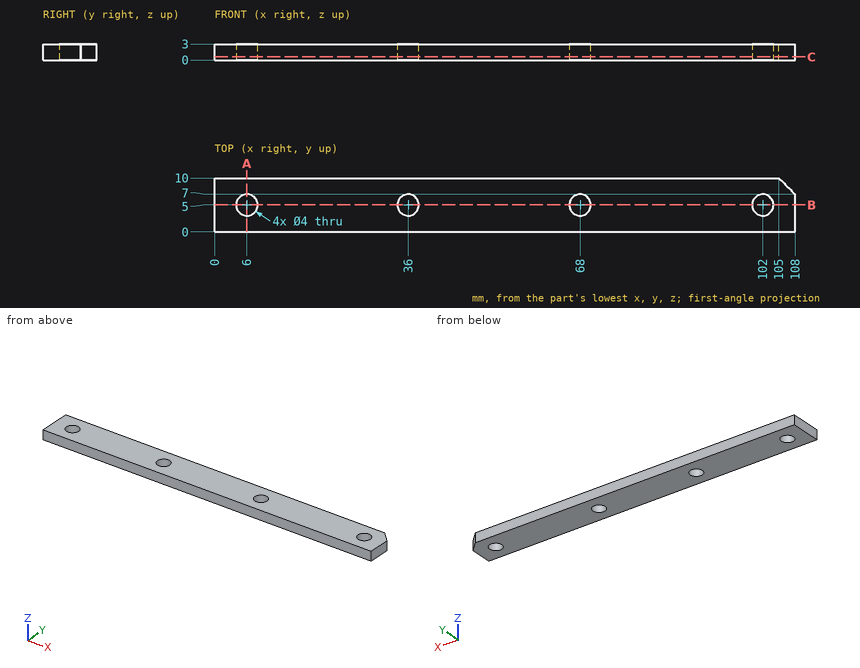
Job drawing, mm, ordinate dimensions from the low corner. One solid piece. Coordinates: 2 decimals unless noted, no trailing zeros. Order: outer loops, then holes, each group sorted by start corner. A loop starts at its lowest first (then second) coordinate and runs counter-clockwise, first axis right, second up. Notation, with made-up numbers: (10.25, 24) -> (17.25, 24) arc R30 cw to (17.25, 63) -> close; hole circle Ø11 at (-24.5, 56.5). An arc over 180 degrees is marked (long way). Put each result on its own line as item: value. Start each with the question number.
(1) Pin check, flat tip, straight feed: pin 1 Ø2.5 at (x, y) = (36, 5) entering from +Z. Stop position of the tip, or through.
(2) Band-saw the part on A-A (x = 6). Give the cut face in (y, z).
(3) Band-saw the part on C-C (z = 0.6). Give the cut face in (x, y), then the cut area to 3 significant figures.
(4) Band-saw the part on B-B (y = 5). Give the cut face in (x, z).
(5) Probe line 1 along X through (y, z) = (5.25, 2.55); line 2 along Y through (x, z) = (6, 2); line 3 along X through (y, z) = (6.5, 2.05). List the from-to ranges inside material, lowest first. Write a range as [from, to].
Determined:
1. pin 1: passes through
2. outline: (0, 0) -> (3, 0) -> (3, 3) -> (0, 3) -> close; (7, 0) -> (10, 0) -> (10, 3) -> (7, 3) -> close
3. outline: (0, 0) -> (108, 0) -> (108, 7) -> (105, 10) -> (0, 10) -> close; hole circle Ø4 at (6, 5); hole circle Ø4 at (36, 5); hole circle Ø4 at (68, 5); hole circle Ø4 at (102, 5)
3. area: 1,030 mm²
4. outline: (0, 0) -> (4, 0) -> (4, 3) -> (0, 3) -> close; (8, 0) -> (34, 0) -> (34, 3) -> (8, 3) -> close; (38, 0) -> (66, 0) -> (66, 3) -> (38, 3) -> close; (70, 0) -> (100, 0) -> (100, 3) -> (70, 3) -> close; (104, 0) -> (108, 0) -> (108, 3) -> (104, 3) -> close
5. line 1: x = [0, 4.02], [7.98, 34.02], [37.98, 66.02], [69.98, 100.02], [103.98, 108]
5. line 2: y = [0, 3], [7, 10]
5. line 3: x = [0, 4.68], [7.32, 34.68], [37.32, 66.68], [69.32, 100.68], [103.32, 108]
